CAD build for the part. Positions are in the model's coordinates, mm. Round coordinates to 2 decimals unless told otherwise and drop trailing zeros. Order: outer loops, then holes, each group sorted by start corner. A loop starts at its lowest first (then second) coordinate and runs counter-clockwise, first axis right, second up. Notation, with made-up numbers: (-7.75, -9) -> (31.25, -9) arc R21 cw to (31.25, 16) -> close; hole circle Ø6 at (78.5, -15.5). An arc over 180 degrees is marked (long way). Answer as CSV lines item,"result". Start each with the question number.
from build123d import *

# Parameters (mm, degrees)
F0_R     = 1.75
F0_R_2   = 1.375
F1_DEPTH = 5.5


with BuildPart() as f1:
    # F0 (on Top) → F1 (new body)
    with BuildSketch(Plane.XY):
        with BuildLine():
            Line((33.2736441009, 20.1755892562), (-24.7263558991, 20.1755892562))
            ThreePointArc((-24.7263558991, 20.1755892562), (-27.2012296333, 19.1504629903), (-28.2263558991, 16.6755892562))
            Line((-28.2263558991, 16.6755892562), (-28.2263558991, -6.3244107438))
            ThreePointArc((-28.2263558991, -6.3244107438), (-27.2012296333, -8.799284478), (-24.7263558991, -9.8244107438))
            Line((-24.7263558991, -9.8244107438), (33.2736441009, -9.8244107438))
            ThreePointArc((33.2736441009, -9.8244107438), (35.748517835, -8.799284478), (36.7736441009, -6.3244107438))
            Line((36.7736441009, -6.3244107438), (36.7736441009, 16.6755892562))
            ThreePointArc((36.7736441009, 16.6755892562), (35.748517835, 19.1504629903), (33.2736441009, 20.1755892562))
        make_face()
        with Locations((-24.7263558991, -6.3244107438)):
            Circle(F0_R, mode=Mode.SUBTRACT)
        with Locations((33.2736441009, -6.3244107438)):
            Circle(F0_R, mode=Mode.SUBTRACT)
        with Locations((-24.7263558991, 16.6755892562)):
            Circle(F0_R, mode=Mode.SUBTRACT)
        with Locations((33.2736441009, 16.6755892562)):
            Circle(F0_R, mode=Mode.SUBTRACT)
        with Locations((-24.7263558991, -6.3244107438)):
            Circle(F0_R)
        with Locations((-24.7263558991, -6.3244107438)):
            Circle(F0_R_2, mode=Mode.SUBTRACT)
        with Locations((-24.7263558991, 16.6755892562)):
            Circle(F0_R)
        with Locations((-24.7263558991, 16.6755892562)):
            Circle(F0_R_2, mode=Mode.SUBTRACT)
        with Locations((33.2736441009, -6.3244107438)):
            Circle(F0_R)
        with Locations((33.2736441009, -6.3244107438)):
            Circle(F0_R_2, mode=Mode.SUBTRACT)
        with Locations((33.2736441009, 16.6755892562)):
            Circle(F0_R)
        with Locations((33.2736441009, 16.6755892562)):
            Circle(F0_R_2, mode=Mode.SUBTRACT)
    extrude(amount=F1_DEPTH)


solid = f1.part
Item 1: Mould opens along X. For faces 1 (the cylindrical face through (34.544, 16.149, 2.712)), 2 (the flat face through (4, 5, 5.5)), 3 (the cylindrical face through (35.72, -8.83, 2.71)) say: released by +X, released by -X, zero draft, split by the parting line, or undercut.
Item 2: Probe line 1 (X direction, y = 16, z = 0.9); line 2 (X direction, y = 15.75, z = 2.5); line 3 (X direction, y = -7.75, z = 3.7). List the from-to ranges inside material, lowest first.
Item 3: Band-saw the part on A-A, the plane z = 2.25. Give the cut face in (x, y) (3 decimals), and give its area (3 significant figures).
Values:
1,face 1,"undercut"
1,face 2,"zero draft"
1,face 3,"released by +X"
2,line 1,"-28.23 to -25.92, -23.53 to 32.08, 34.47 to 36.77"
2,line 2,"-28.23 to -25.74, -23.71 to 32.26, 34.29 to 36.77"
2,line 3,"-27.92 to 36.47"
3,outline,"(-28.226, -6.324) arc R3.5 ccw to (-24.726, -9.824) -> (33.274, -9.824) arc R3.5 ccw to (36.774, -6.324) -> (36.774, 16.676) arc R3.5 ccw to (33.274, 20.176) -> (-24.726, 20.176) arc R3.5 ccw to (-28.226, 16.676) -> close; hole circle Ø2.75 at (-24.726, -6.324); hole circle Ø2.75 at (-24.726, 16.676); hole circle Ø2.75 at (33.274, -6.324); hole circle Ø2.75 at (33.274, 16.676)"
3,area,"1,920 mm²"
